from build123d import *

# Parameters (mm, degrees)
SKETCH1_W                = 48
SKETCH1_H                = 48
SKETCH1_W_2              = 40
SKETCH1_H_2              = 40
BOSS_EXTRUDE1_DEPTH      = 11
SKETCH3_W                = 20
SKETCH3_H                = 6
CUT_EXTRUDE1_DEPTH       = 55.781383699
SKETCH4_W                = 5
SKETCH4_H                = 6
CUT_EXTRUDE2_DEPTH       = 1
SKETCH5_W                = 5
SKETCH5_H                = 6
CUT_EXTRUDE3_DEPTH       = 1
CUT_EXTRUDE4_REACH       = 56.781
SKETCH6_R                = 1.35
CUT_EXTRUDE5_REACH       = 56.781
SKETCH7_R                = 1.35
CUT_EXTRUDE6_REACH       = 56.781
SKETCH8_R                = 1.35
CUT_EXTRUDE7_REACH       = 56.781
SKETCH9_R                = 1.65
BOSS_EXTRUDE7_DEPTH      = 8
BOSS_EXTRUDE7_DEPTH_BACK = 10


with BuildPart() as part:
    # Sketch1 → Boss-Extrude1 (new body)
    with BuildSketch(Plane(origin=(0, 0, 0), x_dir=(1, 0, 0), z_dir=(0, 1, 0))):
        Rectangle(SKETCH1_W, SKETCH1_H)
        Rectangle(SKETCH1_W_2, SKETCH1_H_2, mode=Mode.SUBTRACT)
    extrude(amount=BOSS_EXTRUDE1_DEPTH)

    # Sketch3 → Cut-Extrude1 (cut, through all)
    with BuildSketch(Plane.XY.offset(24)):
        with Locations((0, 3)):
            Rectangle(SKETCH3_W, SKETCH3_H)
    extrude(amount=-CUT_EXTRUDE1_DEPTH, mode=Mode.SUBTRACT)

    # Sketch4 → Cut-Extrude2 (cut)
    with BuildSketch(Plane.XY.offset(-20)):
        with Locations((-12.5, 3)):
            Rectangle(SKETCH4_W, SKETCH4_H)
        with Locations((12.5, 3)):
            Rectangle(SKETCH4_W, SKETCH4_H)
    extrude(amount=-CUT_EXTRUDE2_DEPTH, mode=Mode.SUBTRACT)

    # Sketch5 → Cut-Extrude3 (cut)
    with BuildSketch(Plane(origin=(0, 0, 20), x_dir=(-1, 0, 0), z_dir=(0, 0, -1))):
        with Locations((-12.5, 3)):
            Rectangle(SKETCH5_W, SKETCH5_H)
        with Locations((12.5, 3)):
            Rectangle(SKETCH5_W, SKETCH5_H)
    extrude(amount=-CUT_EXTRUDE3_DEPTH, mode=Mode.SUBTRACT)

    # Sketch6 → Cut-Extrude4 (cut, up to next)
    with BuildSketch(Plane(origin=(0, 0, -24), x_dir=(-1, 0, 0), z_dir=(0, 0, -1)), mode=Mode.PRIVATE) as cut_extrude4_sk1:
        with Locations((-9, 9)):
            Circle(SKETCH6_R)
    cut_extrude4_tool1 = extrude(cut_extrude4_sk1.sketch, amount=-CUT_EXTRUDE4_REACH, mode=Mode.PRIVATE) & part.part
    # Sketch6 → Cut-Extrude4 (cut, up to next)
    with BuildSketch(Plane(origin=(0, 0, -24), x_dir=(-1, 0, 0), z_dir=(0, 0, -1)), mode=Mode.PRIVATE) as cut_extrude4_sk2:
        with Locations((9, 9)):
            Circle(SKETCH6_R)
    cut_extrude4_tool2 = extrude(cut_extrude4_sk2.sketch, amount=-CUT_EXTRUDE4_REACH, mode=Mode.PRIVATE) & part.part
    add(cut_extrude4_tool1.solids().sort_by_distance((9, 9, -24))[0], mode=Mode.SUBTRACT)
    add(cut_extrude4_tool2.solids().sort_by_distance((-9, 9, -24))[0], mode=Mode.SUBTRACT)

    # Sketch7 → Cut-Extrude5 (cut, up to next)
    with BuildSketch(Plane.XY.offset(24), mode=Mode.PRIVATE) as cut_extrude5_sk1:
        with Locations((9.5, 8.412816521)):
            Circle(SKETCH7_R)
    cut_extrude5_tool1 = extrude(cut_extrude5_sk1.sketch, amount=-CUT_EXTRUDE5_REACH, mode=Mode.PRIVATE) & part.part
    # Sketch7 → Cut-Extrude5 (cut, up to next)
    with BuildSketch(Plane.XY.offset(24), mode=Mode.PRIVATE) as cut_extrude5_sk2:
        with Locations((-5.5, 8.412816521)):
            Circle(SKETCH7_R)
    cut_extrude5_tool2 = extrude(cut_extrude5_sk2.sketch, amount=-CUT_EXTRUDE5_REACH, mode=Mode.PRIVATE) & part.part
    add(cut_extrude5_tool1.solids().sort_by_distance((9.5, 8.412817, 24))[0], mode=Mode.SUBTRACT)
    add(cut_extrude5_tool2.solids().sort_by_distance((-5.5, 8.412817, 24))[0], mode=Mode.SUBTRACT)

    # Sketch8 → Cut-Extrude6 (cut, up to next)
    with BuildSketch(Plane(origin=(24, 0, 0), x_dir=(0, 0, -1), z_dir=(1, 0, 0)), mode=Mode.PRIVATE) as cut_extrude6_sk1:
        with Locations((-12, 4)):
            Circle(SKETCH8_R)
    cut_extrude6_tool1 = extrude(cut_extrude6_sk1.sketch, amount=-CUT_EXTRUDE6_REACH, mode=Mode.PRIVATE) & part.part
    # Sketch8 → Cut-Extrude6 (cut, up to next)
    with BuildSketch(Plane(origin=(24, 0, 0), x_dir=(0, 0, -1), z_dir=(1, 0, 0)), mode=Mode.PRIVATE) as cut_extrude6_sk2:
        with Locations((-6.5, 4)):
            Circle(SKETCH8_R)
    cut_extrude6_tool2 = extrude(cut_extrude6_sk2.sketch, amount=-CUT_EXTRUDE6_REACH, mode=Mode.PRIVATE) & part.part
    # Sketch8 → Cut-Extrude6 (cut, up to next)
    with BuildSketch(Plane(origin=(24, 0, 0), x_dir=(0, 0, -1), z_dir=(1, 0, 0)), mode=Mode.PRIVATE) as cut_extrude6_sk3:
        with Locations(Location((6.5, 4, 0), (0, 0, 180))):
            Circle(SKETCH8_R)
    cut_extrude6_tool3 = extrude(cut_extrude6_sk3.sketch, amount=-CUT_EXTRUDE6_REACH, mode=Mode.PRIVATE) & part.part
    # Sketch8 → Cut-Extrude6 (cut, up to next)
    with BuildSketch(Plane(origin=(24, 0, 0), x_dir=(0, 0, -1), z_dir=(1, 0, 0)), mode=Mode.PRIVATE) as cut_extrude6_sk4:
        with Locations(Location((12, 4, 0), (0, 0, 180))):
            Circle(SKETCH8_R)
    cut_extrude6_tool4 = extrude(cut_extrude6_sk4.sketch, amount=-CUT_EXTRUDE6_REACH, mode=Mode.PRIVATE) & part.part
    add(cut_extrude6_tool1.solids().sort_by_distance((24, 4, 12))[0], mode=Mode.SUBTRACT)
    add(cut_extrude6_tool2.solids().sort_by_distance((24, 4, 6.5))[0], mode=Mode.SUBTRACT)
    add(cut_extrude6_tool3.solids().sort_by_distance((24, 4, -6.5))[0], mode=Mode.SUBTRACT)
    add(cut_extrude6_tool4.solids().sort_by_distance((24, 4, -12))[0], mode=Mode.SUBTRACT)

    # Sketch9 → Cut-Extrude7 (cut, up to next)
    with BuildSketch(Plane.ZY.offset(24), mode=Mode.PRIVATE) as cut_extrude7_sk1:
        with Locations((0, 6)):
            Circle(SKETCH9_R)
    cut_extrude7_tool1 = extrude(cut_extrude7_sk1.sketch, amount=-CUT_EXTRUDE7_REACH, mode=Mode.PRIVATE) & part.part
    add(cut_extrude7_tool1.solids().sort_by_distance((-24, 6, 0))[0], mode=Mode.SUBTRACT)

    # Sketch10 → Boss-Extrude7 (add, two sides: drawn at the far end of the back side and taken through both)
    with BuildSketch(Plane(origin=(24, 0, 0), x_dir=(0, 0, -1), z_dir=(1, 0, 0)).offset(-BOSS_EXTRUDE7_DEPTH_BACK)):
        with BuildLine():
            Line((-42, 0), (-20, 0))
            Line((-20, 0), (-20, 11))
            Line((-20, 11), (-25.711810571, 21.622325672))
            ThreePointArc((-25.711810571, 21.622325672), (-32.713932588, 5.745809356), (-46.4, 16.412816521))
            Line((-46.4, 16.412816521), (-46.4, 8.182735119))
            Line((-46.4, 8.182735119), (-42, 0))
        make_face()
        with BuildLine():
            ThreePointArc((-46.4, 16.412816521), (-32.713932588, 5.745809356), (-25.711810571, 21.622325672))
            Line((-25.711810571, 21.622325672), (-26.592555065, 21.148733931))
            ThreePointArc((-26.592555065, 21.148733931), (-32.958120534, 6.71553728), (-45.4, 16.412816521))
            Line((-45.4, 16.412816521), (-46.4, 16.412816521))
        make_face()
    extrude(amount=BOSS_EXTRUDE7_DEPTH + BOSS_EXTRUDE7_DEPTH_BACK)


solid = part.part
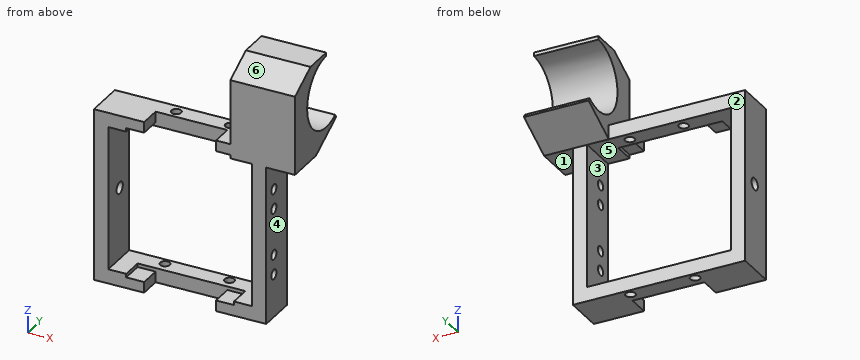
Work out the finished part from the listing and answer in its coordinate system (mm). Face numbers are marked on the shaded views. A direction names the side the tool comes from. Round coordinates to 2 decimals unless told otherwise and drop trailing zeros. Write each loop counter-clockwise with the first axis right and the second up, starting at its lowest first coordinate (ties: lowest second). Pieces come first, ordered by that corner, then holes. Notation, with made-up numbers: M 32,39.5 L 90,39.5 A11 ccw 90,59.5 Z; hole C 36,-13 d5. An arc over 180 degrees is marked long. Use a Markdown table: item, result.
1) The part is cut by section C-C on z = -6.5. Give the vertices of the cut face in (x, y).
Taken from the geometry:
| item | result |
|---|---|
| outline | M -24,0 L -20,0 L -20,11 L -24,11 Z; M 20,0 L 24,0 L 24,2.65 L 20,2.65 Z; M 20,5.35 L 24,5.35 L 24,11 L 20,11 Z |
2) The part is cut by section D-D on y = 14.25. Give the vertices of the cut face in (x, z), plus the area to 3 significant figures.
Taken from the geometry:
| item | result |
|---|---|
| outline | M 14,21.75 L 32,21.75 L 32,25.64 L 14,25.64 Z; M 14,45.16 L 32,45.16 L 32,46.4 L 14,46.4 Z |
| area | 92.3 mm2 |
3) Which of the six approach directions +Z, -Z, +X, -X, +Y, -Y give full straight-line access (tool end or side, diameter ignored) to the marked faces 1, 2 and 3?
Taken from the geometry:
| item | result |
|---|---|
| face 1 | -Z, +X, +Y, -Y |
| face 2 | -Z, -X, +Y |
| face 3 | +Y, -Y |
4) The part is cut by section A-A on z = 4. Give the vertices of the cut face in (x, y).
Taken from the geometry:
| item | result |
|---|---|
| outline | M -24,0 L -20,0 L -20,11 L -24,11 Z; M 20,0 L 24,0 L 24,11 L 20,11 Z |
5) Flat-ended cylindrical pins translate along their axes: pin 1 (4.5 mm diameter, centred on x = -9, y = 9, fed in from +Z); pin 2 (9 mm diameter, centred on y = 5.5, z = 9, fed in from +X); pin 3 (24 mm diameter, centred on x = 7.5, z = -10.5, fed in from +Y). Find the tip coordinate at first contact, or state that the pin passes through.
Taken from the geometry:
| item | result |
|---|---|
| pin 1 | stops at z = 24 |
| pin 2 | stops at x = 24 |
| pin 3 | stops at y = 11 |
6) Consider line 1 (X direction, y = 2.5, z = -15.5); line 2 (Y direction, x = -9, z = -23.15). Determine where each line is inside the solid, lowest interval first. Write a range as [from, to].
Taken from the geometry:
| item | result |
|---|---|
| line 1 | x = [-24, -20], [20, 24] |
| line 2 | y = [6, 7.65], [10.35, 11] |
7) Determine the mould class of the marked faces 4, 5 and 6 for opening direction Z: pulls with the +Z half, pulls with the -Z half, needs draft (parallel to the pull), parting line crosses it, or undercut.
Taken from the geometry:
| item | result |
|---|---|
| face 4 | needs draft |
| face 5 | undercut |
| face 6 | pulls with the +Z half |
8) The part is cut by section B-B on x = 16.5. Give the vertices of the cut face in (y, z).
Taken from the geometry:
| item | result |
|---|---|
| outline | M 0,-24 L 11,-24 L 11,-20 L 0,-20 Z; M 0,20 L 11,20 L 21.62,25.71 L 21.15,26.59 A10 cw long 16.41,45.4 L 16.41,46.4 L 8.18,46.4 L 0,42 Z |
